```python
from build123d import *

# Parameters (mm, degrees)
F1_DEPTH = 2
F3_DEPTH = 7
F4_R     = 0.6
F5_R     = 4
F6_R     = 1


# Not quite as in the source:
# - a feature of the source that left no trace in its solid (it failed there, or was rolled back) is left out


with BuildPart() as f1:
    # F0 (on Top) → F1 (new body)
    with BuildSketch(Plane.XY):
        Polygon((0, 12.3), (0, 0), (70, 0), (70, 9.5), align=None)
    extrude(amount=F1_DEPTH)

    # F2 (on face) → F3 (join)
    with BuildSketch(Plane.XY.offset(2)):
        Polygon((1, 11.8), (1, 8.8), (7.8769936128, 8.5249202555), (10.9920095872, 11.4003196165), align=None)
        Polygon((63.4, 7.0580007994), (69.9, 9.3), (49.9159808256, 10.099360767), (57.8044746312, 7.2818218141), align=None)
    extrude(amount=-F3_DEPTH)

    # F4
    f4_edges = [f1.edges().sort_by_distance(p)[0] for p in [
        (1, 11.8, -2.5),
        (10.99201, 11.40032, -2.5),
        (69.9, 9.3, -2.5),
        (49.915981, 10.099361, -2.5),
        (63.4, 7.058001, -2.5),
        (57.804475, 7.281822, -2.5),
        (1, 8.8, -2.5),
        (7.876994, 8.52492, -2.5),
    ]]
    fillet(f4_edges, radius=F4_R)

    # F5
    f5_edges = [f1.edges().sort_by_distance(p)[0] for p in [
        (70, 9.5, 1),
    ]]
    fillet(f5_edges, radius=F5_R)

    # F6
    f6_edges = [f1.edges().sort_by_distance(p)[0] for p in [
        (0, 12.3, 1),
    ]]
    fillet(f6_edges, radius=F6_R)


solid = f1.part
```
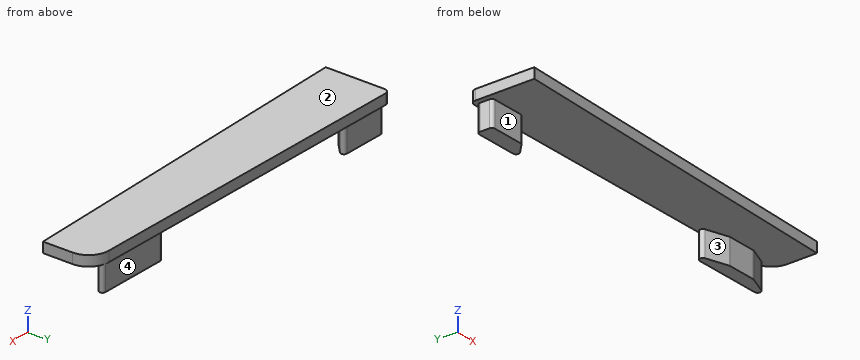
The listing builds one solid part. Answer for the finished solid, in the listing's coordinates (mm). Face numbers are marked on the shaded views. A direction names the side the tool comes from. Round coordinates to 2 decimals unless told otherwise and drop trailing zeros. Loops run counter-clockwise (first coordinate to the right, second up) from the corner with the lowest first, then second, coordinate; pieces in that order, holes last. Notation, with made-up numbers: (12.5, 8.5) - (42.5, 8.5) arc R31 cw to (42.5, 37.5) - close; hole circle Ø2 at (70, 79.5). An arc over 180 degrees is marked (long way). Return JSON: item names as keys, results as strings. Group by question number.
1. Consider probe 1 along Z at (x, y) = (18.5, 9); probe 2 along Y at (x, z) = (13.5, 1); probe 3 along Y at (x, z) = (63.5, -1.5). Determine where each line is inside the solid, lowest interval first.
2. The part is cut by section A-A on z = -2.25. Determine the outline of the cut face in (x, y).
3. Each of these flat-tipped pins is pushed along its axis until it touches: P1, Ø1.4, axis at y = 10, z = -3.5, coming from the -X side; P2, Ø1, axis at x = 56, y = 11, coming from the -Z side; P3, Ø2, axis at x = 61.5, z = -3.5, coming from the +Y side. Where does it stop, or does it pass through?
4. The part is cut by section C-C on z = 1. Determine the outline of the cut face in (x, y), then the cut area to 3 significant figures.
5. Which of the six approach directions +Z, -Z, +X, -X, +Y, -Y give full straight-line access (tool end or side, diameter ignored) to the marked faces 1, 2, 3 and 4?
6. The part is cut by section B-B on x = 5.5. Determine the outline of the cut face in (y, z).
7. The part is cut by section D-D on y = 4.5. Determine the outline of the cut face in (x, z).
Resolved:
{
 "1": {"probe 1": "z = 0 to 2", "probe 2": "y = 0 to 11.76", "probe 3": "y = 7.09 to 9.56"},
 "2": {"outline": "(1, 9.38) arc R0.6 ccw to (1.58, 8.78) - (7.63, 8.53) arc R0.6 ccw to (8.06, 8.69) - (9.93, 10.42) arc R0.6 ccw to (9.54, 11.46) - (1.62, 11.78) arc R0.6 ccw to (1, 11.18) - close; (53.62, 8.78) - (57.72, 7.31) arc R0.6 ccw to (57.9, 7.28) - (63.29, 7.06) arc R0.6 ccw to (63.51, 7.09) - (66.89, 8.26) arc R0.6 ccw to (66.72, 9.43) - (53.84, 9.94) arc R0.6 ccw to start"},
 "3": {"P1": "stops at x = 1", "P2": "passes through", "P3": "stops at y = 9.68"},
 "4": {"outline": "(0, 0) - (70, 0) - (70, 5.66) arc R4 ccw to (66.16, 9.65) - (1.04, 12.26) arc R1 ccw to (0, 11.26) - close", "area": "760 mm²"},
 "5": {"face 1": "-Z, -X, -Y", "face 2": "+Z, +X, -X, +Y, -Y", "face 3": "-Z, -Y", "face 4": "-Z, +X, +Y"},
 "6": {"outline": "(0, 0) - (8.62, 0) - (8.62, -5) - (11.62, -5) - (11.62, 0) - (12.08, 0) - (12.08, 2) - (0, 2) - close"},
 "7": {"outline": "(0, 0) - (70, 0) - (70, 2) - (0, 2) - close"}
}
